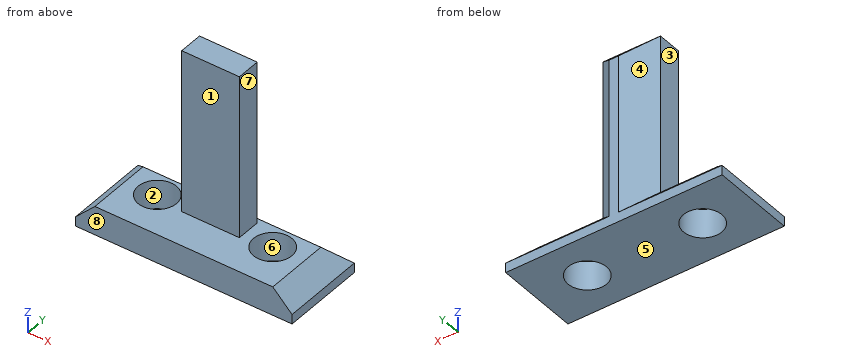
```python
from build123d import *

# Parameters (mm, degrees)
SKETCH1_W           = 22.5
SKETCH1_H           = 8.75
SKETCH1_R           = 2
BOSS_EXTRUDE1_DEPTH = 3
SKETCH2_W           = 3
SKETCH2_H           = 17
BOSS_EXTRUDE2_DEPTH = 5
CHAMFER1_SIZE       = 2
CHAMFER2_SIZE       = 2.5


with BuildPart() as part:
    # Sketch1 → Boss-Extrude1 (new body)
    with BuildSketch(Plane.XY):
        Rectangle(SKETCH1_W, SKETCH1_H)
        with Locations((6, 0)):
            Circle(SKETCH1_R, mode=Mode.SUBTRACT)
        with Locations(Location((-6, 0, 0), (0, 0, 180))):
            Circle(SKETCH1_R, mode=Mode.SUBTRACT)
    extrude(amount=BOSS_EXTRUDE1_DEPTH)

    # Sketch2 → Boss-Extrude2 (add)
    with BuildSketch(Plane(origin=(0, 4.375, 0), x_dir=(1, 0, 0), z_dir=(0, 1, 0))):
        with Locations((-1.5, -11.5)):
            Rectangle(SKETCH2_W, SKETCH2_H)
        with Locations((1.5, -11.5)):
            Rectangle(SKETCH2_W, SKETCH2_H)
    extrude(amount=-BOSS_EXTRUDE2_DEPTH)

    # Chamfer1
    chamfer1_edges = [part.edges().sort_by_distance(p)[0] for p in [
        (-11.25, 0, 3),
        (-7.125, 4.375, 3),
        (11.25, 0, 3),
        (7.125, 4.375, 3),
    ]]
    chamfer(chamfer1_edges, length=CHAMFER1_SIZE)

    # Chamfer2
    # the kernel refuses this chamfer: 2.5 mm, written as the material it takes off along each edge
    with BuildSketch(Plane(origin=(3, 4.375, 26.42920747), x_dir=(0.027495876610586317, -0.9996219169112968, 0), z_dir=(0, 0, -1))) as chamfer2_piece_1_section:
        Polygon((CHAMFER2_SIZE * 0.999621916911, CHAMFER2_SIZE * 0.0274958766106), (-CHAMFER2_SIZE * 0.0274958766106, CHAMFER2_SIZE * 0.999621916911), (0, 0), align=None)
    chamfer2_piece_1 = extrude(amount=31.85841494, mode=Mode.PRIVATE)
    chamfer2_piece_1 = split(chamfer2_piece_1, bisect_by=Plane(origin=(2.16638878, 3.54222244, 3), z_dir=(0, 0, 1)), keep=Keep.TOP, mode=Mode.PRIVATE)
    add(chamfer2_piece_1, mode=Mode.SUBTRACT)
    with BuildSketch(Plane(origin=(3, 4.375, 26.42920747), x_dir=(0.027495876610586317, -0.9996219169112968, 0), z_dir=(0, 0, -1))) as chamfer2_piece_2_section:
        Polygon((CHAMFER2_SIZE * 0.999621916911, CHAMFER2_SIZE * 0.0274958766106), (-CHAMFER2_SIZE * 0.0274958766106, CHAMFER2_SIZE * 0.999621916911), (0, 0), align=None)
    chamfer2_piece_2 = extrude(amount=31.85841494, mode=Mode.PRIVATE)
    chamfer2_piece_2 = split(chamfer2_piece_2, bisect_by=Plane(origin=(2.022727273, 3.465909091, 1.909090909), z_dir=(0, 0.7071067811865476, 0.7071067811865476)), keep=Keep.TOP, mode=Mode.PRIVATE)
    add(chamfer2_piece_2, mode=Mode.SUBTRACT)
    with BuildSketch(Plane(origin=(9.42920747, 4.375, 20), x_dir=(0, -0.9996219169112968, 0.027495876610586317), z_dir=(-1, 0, 0))) as chamfer2_piece_3:
        Polygon((CHAMFER2_SIZE * 0.999621916911, -CHAMFER2_SIZE * 0.0274958766106), (-CHAMFER2_SIZE * 0.0274958766106, -CHAMFER2_SIZE * 0.999621916911), (0, 0), align=None)
    extrude(amount=18.85841494, mode=Mode.SUBTRACT)
    with BuildSketch(Plane(origin=(-3, 4.375, -5.42920747), x_dir=(-0.027495876610586147, -0.9996219169112968, 0), z_dir=(0, 0, 1))) as chamfer2_piece_4_section:
        Polygon((CHAMFER2_SIZE * 0.999621916911, CHAMFER2_SIZE * 0.0274958766106), (-CHAMFER2_SIZE * 0.0274958766106, CHAMFER2_SIZE * 0.999621916911), (0, 0), align=None)
    chamfer2_piece_4 = extrude(amount=31.85841494, mode=Mode.PRIVATE)
    chamfer2_piece_4 = split(chamfer2_piece_4, bisect_by=Plane(origin=(-2.022727273, 3.465909091, 1.909090909), z_dir=(0, 0.7071067811865476, 0.7071067811865476)), keep=Keep.TOP, mode=Mode.PRIVATE)
    add(chamfer2_piece_4, mode=Mode.SUBTRACT)
    with BuildSketch(Plane(origin=(-3, 4.375, -5.42920747), x_dir=(-0.027495876610586147, -0.9996219169112968, 0), z_dir=(0, 0, 1))) as chamfer2_piece_5_section:
        Polygon((CHAMFER2_SIZE * 0.999621916911, CHAMFER2_SIZE * 0.0274958766106), (-CHAMFER2_SIZE * 0.0274958766106, CHAMFER2_SIZE * 0.999621916911), (0, 0), align=None)
    chamfer2_piece_5 = extrude(amount=31.85841494, mode=Mode.PRIVATE)
    chamfer2_piece_5 = split(chamfer2_piece_5, bisect_by=Plane(origin=(-2.875, 2.125, 3), z_dir=(0, 0, 1)), keep=Keep.TOP, mode=Mode.PRIVATE)
    add(chamfer2_piece_5, mode=Mode.SUBTRACT)


solid = part.part
```
Input: part model. Units: mm. Frame: model coordinates. Face numbers are marked on the shaded views. A direction names the side the tool comes from. Give positions to 0.01 mm unless a question says otherwise; leave off trailing zeros. Loops run counter-clockwise (first coordinate to the right, second up) from the corner with the lowest first, then second, coordinate; pieces in that order, holes last. Notation, with made-up numbers: (-29.5, 14) -> (-20.5, 14) arc R9 ccw to (-20.5, 25) -> close; hole circle Ø7 at (-21.5, -37). An arc over 180 degrees is marked (long way). Use a Markdown table: item, result.
Q1. Section query D-D, the plane y = -3.25. Return the cut outline in (x, z), plus the area to 3 significant figures.
Entries:
| item | result |
|---|---|
| outline | (-11.25, 0) -> (11.25, 0) -> (11.25, 1) -> (9.25, 3) -> (-9.25, 3) -> (-11.25, 1) -> close |
| area | 63.5 mm² |
Q2. First-contact query: P1, Ø4.5, axis at x = -6, y = 0, coming from the +Z side; P2, Ø3, axis at y = 0, z = 15, coming from the +X side; P3, Ø0.8, axis at y = 0, z = 10, coming from the -X side. Flat tips, straight axial feed; report the tip coordinate or a pass-through.
Entries:
| item | result |
|---|---|
| P1 | stops at z = 3 |
| P2 | stops at x = 3 |
| P3 | stops at x = -3 |
Q3. Access query for the marked faces 1, 2, 3, 4 and 5. Directions: +Z, -Z, +X, -X, +Y, -Y. A direction counts if a zero-diameter tool reaches every point of the face in a straight line with its end or side. Return the directions, or none.
Entries:
| item | result |
|---|---|
| face 1 | +Z, +X, -X, -Y |
| face 2 | +Z, -Z |
| face 3 | +Z, -X, +Y, -Y |
| face 4 | +Z, -X, +Y |
| face 5 | -Z, +X, -X, +Y, -Y |
Q4. Section query C-C, the plane z = 10.5. Return the cut outline in (x, y) (3 decimals).
Entries:
| item | result |
|---|---|
| outline | (-3, -0.625) -> (3, -0.625) -> (3, 1.875) -> (0.5, 4.375) -> (-0.5, 4.375) -> (-3, 1.875) -> close |
Q5. Section query A-A, the plane x = -6. Return the cut outline in (y, z) (3 decimals), plus the area to 4 significant figures.
Entries:
| item | result |
|---|---|
| outline | (-4.375, 0) -> (-2, 0) -> (-2, 3) -> (-4.375, 3) -> close; (2, 0) -> (4.375, 0) -> (4.375, 1) -> (2.375, 3) -> (2, 3) -> close |
| area | 12.25 mm² |
Q6. Ray query, probe 1 along Y at (x, z) = (6, 0.85) (3 decimals); probe 2 along Z at (x, y) = (4, -2); probe 3 along Y at (x, z) = (6, 2.3) (3 decimals). Return the intervals inside material, ascending. Write a range as from..to.
Entries:
| item | result |
|---|---|
| probe 1 | y = -4.375..-2, 2..4.375 |
| probe 2 | z = 0..3 |
| probe 3 | y = -4.375..-2, 2..3.075 |
Q7. Section query B-B, the plane y = 0. Return the cut outline in (x, z).
Entries:
| item | result |
|---|---|
| outline | (-11.25, 0) -> (-8, 0) -> (-8, 3) -> (-9.25, 3) -> (-11.25, 1) -> close; (-4, 0) -> (4, 0) -> (4, 3) -> (3, 3) -> (3, 20) -> (-3, 20) -> (-3, 3) -> (-4, 3) -> close; (8, 0) -> (11.25, 0) -> (11.25, 1) -> (9.25, 3) -> (8, 3) -> close |
Q8. Pull-direction query (Y, two-part tool) for the marked faces 6, 7 and 8; classes: pulls with the +Y half, pulls with the -Y half, needs draft (parallel to the pull), parting line crosses it, or undercut.
Entries:
| item | result |
|---|---|
| face 6 | undercut |
| face 7 | needs draft |
| face 8 | pulls with the -Y half |
